Geometry check sheet. Reference: the model listing, model coordinates, mm. A direction names the side the tool comes from. Coordinates: 2 decimals unless noted, no trailing zeros. Write each loop counter-clockwise with the first axis right and the second up, starting at its lowest first coordinate (ties: lowest second). Pieces come first, ordered by that corner, then holes. Notation, with made-up numbers: (-37.5, 83) -> (-32.5, 83) arc R26 ccw to (-32.5, 116) -> close; hole circle Ø9 at (-16, -32). An arc over 180 degrees is marked (long way). Use a Markdown table: item, result.
```python
from build123d import *

# Parameters (mm, degrees)
ESQUISSE1_W             = 45
ESQUISSE1_H             = 18
EXTRUSION1_DEPTH        = 2
CONG_1_R                = 3
ENL_V_MAT_EXTRU_1_REACH = 4
ESQUISSE2_R             = 3.5


with BuildPart() as part:
    # Esquisse1 → Extrusion1 (new body)
    with BuildSketch(Plane.XY):
        Rectangle(ESQUISSE1_W, ESQUISSE1_H)
    extrude(amount=EXTRUSION1_DEPTH)

    # Congé1
    cong_1_edges = [part.edges().sort_by_distance(p)[0] for p in [
        (-22.5, 9, 1),
        (22.5, 9, 1),
        (22.5, -9, 1),
        (-22.5, -9, 1),
    ]]
    fillet(cong_1_edges, radius=CONG_1_R)

    # Esquisse2 → Enlèv. mat.-Extru.1 (cut, up to next)
    with BuildSketch(Plane.XY.offset(2), mode=Mode.PRIVATE) as enl_v_mat_extru_1_sk1:
        Circle(ESQUISSE2_R)
    enl_v_mat_extru_1_tool1 = extrude(enl_v_mat_extru_1_sk1.sketch, amount=-ENL_V_MAT_EXTRU_1_REACH, mode=Mode.PRIVATE) & part.part
    add(enl_v_mat_extru_1_tool1.solids().sort_by_distance((0, 0, 2))[0], mode=Mode.SUBTRACT)
    # Esquisse2 → Enlèv. mat.-Extru.1 (cut, up to next)
    with BuildSketch(Plane.XY.offset(2), mode=Mode.PRIVATE) as enl_v_mat_extru_1_sk2:
        with BuildLine():
            Line((17, 2), (19, 2))
            ThreePointArc((19, 2), (21, 0), (19, -2))
            Line((19, -2), (17, -2))
            ThreePointArc((17, -2), (15, 0), (17, 2))
        make_face()
    enl_v_mat_extru_1_tool2 = extrude(enl_v_mat_extru_1_sk2.sketch, amount=-ENL_V_MAT_EXTRU_1_REACH, mode=Mode.PRIVATE) & part.part
    add(enl_v_mat_extru_1_tool2.solids().sort_by_distance((18, 0, 2))[0], mode=Mode.SUBTRACT)
    # Esquisse2 → Enlèv. mat.-Extru.1 (cut, up to next)
    with BuildSketch(Plane.XY.offset(2), mode=Mode.PRIVATE) as enl_v_mat_extru_1_sk3:
        with BuildLine():
            Line((-19, -2), (-17, -2))
            ThreePointArc((-17, -2), (-15, 0), (-17, 2))
            Line((-17, 2), (-19, 2))
            ThreePointArc((-19, 2), (-21, 0), (-19, -2))
        make_face()
    enl_v_mat_extru_1_tool3 = extrude(enl_v_mat_extru_1_sk3.sketch, amount=-ENL_V_MAT_EXTRU_1_REACH, mode=Mode.PRIVATE) & part.part
    add(enl_v_mat_extru_1_tool3.solids().sort_by_distance((-18, 0, 2))[0], mode=Mode.SUBTRACT)


solid = part.part
```
Item 1: Section check C-C on y = 0. Record the boundary of the cut face in (x, z), then the cut area to 3 significant figures.
Answer block:
| item | result |
|---|---|
| outline | (-22.5, 0) -> (-21, 0) -> (-21, 2) -> (-22.5, 2) -> close; (-15, 0) -> (-3.5, 0) -> (-3.5, 2) -> (-15, 2) -> close; (3.5, 0) -> (15, 0) -> (15, 2) -> (3.5, 2) -> close; (21, 0) -> (22.5, 0) -> (22.5, 2) -> (21, 2) -> close |
| area | 52.0 mm^2 |
Item 2: Mould release check, pull along Y, two halves, no side actions. Record for faces 1 (the cylindrical face through (-21.64, -8.1, 1.01)), 2 (the flat face through (0, 4, 2)), 3 (the flat face through (-18, -2, 1)): +Y half, -Y half, draft (parallel to the pull), parting line (faces both ways), or undercut.
Answer block:
| item | result |
|---|---|
| face 1 | -Y half |
| face 2 | draft |
| face 3 | undercut |
Item 3: Tool access check on faces 4 (the cylindrical face through (21, 0, 1)), 5 (the flat face through (0, -9, 1)). Record the directions out of +Z, -Z, +X, -X, +Y, -Y that give a thin tool (end or side, any length) a straight path to the whole face; none if there is none.
Answer block:
| item | result |
|---|---|
| face 4 | +Z, -Z |
| face 5 | +Z, -Z, +X, -X, -Y |
Item 4: Section check A-A on z = 1.35. Record the boundary of the cut face in (x, y).
Answer block:
| item | result |
|---|---|
| outline | (-22.5, -6) arc R3 ccw to (-19.5, -9) -> (19.5, -9) arc R3 ccw to (22.5, -6) -> (22.5, 6) arc R3 ccw to (19.5, 9) -> (-19.5, 9) arc R3 ccw to (-22.5, 6) -> close; hole (-19, -2) -> (-17, -2) arc R2 ccw to (-17, 2) -> (-19, 2) arc R2 ccw to start; hole circle Ø7 at (0, 0); hole (17, -2) -> (19, -2) arc R2 ccw to (19, 2) -> (17, 2) arc R2 ccw to start |
Item 5: Section check D-D on y = 3. Record the boundary of the cut face in (x, z).
Answer block:
| item | result |
|---|---|
| outline | (-22.5, 0) -> (-1.8, 0) -> (-1.8, 2) -> (-22.5, 2) -> close; (1.8, 0) -> (22.5, 0) -> (22.5, 2) -> (1.8, 2) -> close |
Item 6: Thickness scan on L1, parallel to Y at x = 0, z = 0.6; L2, parallel to Y at x = -16.5, z = 0.7; L3, parallel to X at y = -6.25, z = 0.1. Record the ranges inside material, lowest first. Write a range as [from, to].
Answer block:
| item | result |
|---|---|
| L1 | y = [-9, -3.5], [3.5, 9] |
| L2 | y = [-9, -1.94], [1.94, 9] |
| L3 | x = [-22.49, 22.49] |
Item 7: Section check B-B on x = 2. Record the boundary of the cut face in (y, z), then the cut area to 3 significant figures.
Answer block:
| item | result |
|---|---|
| outline | (-9, 0) -> (-2.87, 0) -> (-2.87, 2) -> (-9, 2) -> close; (2.87, 0) -> (9, 0) -> (9, 2) -> (2.87, 2) -> close |
| area | 24.5 mm^2 |
